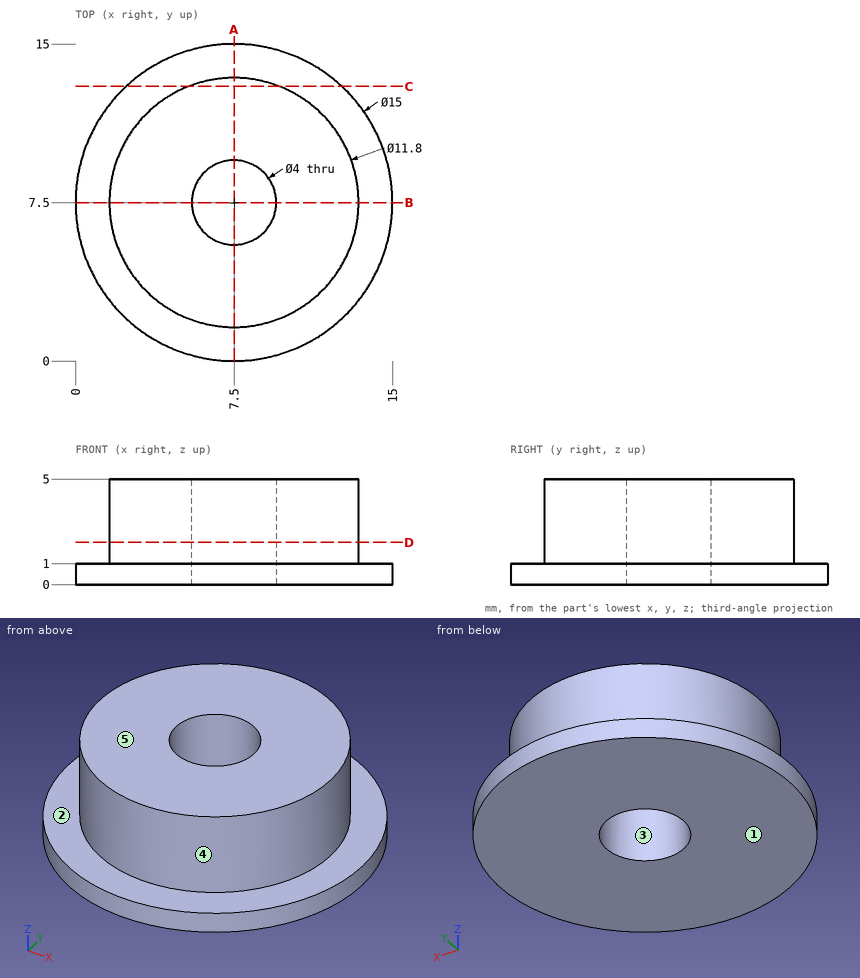
For this review, use the dimensioned drawing (mm, ordinates from the lowest corner) and the shaded views. A direction names the side the tool comes from. Coordinates: 2 decimals unless noted, no trailing zeros. Loops run counter-clockwise (first coordinate to the right, second up) from the corner with the lowest first, then second, coordinate; pieces in that order, holes last. Notation, with made-up numbers: (55.25, 64) -> (112.25, 64) arc R22 ccw to (112.25, 92) -> close; hole circle Ø6 at (79, -24.75). An arc over 180 degrees is marked (long way). Use a Markdown table: item, result. Add a question column.
1. To check wall thickness, follow line 1 (Y direction, x = 7.5, z = 2.75); line 2 (Z direction, x = 11.75, y = 13); line 3 (X direction, y = 5.75, z = 3.1). State the ranges of each line that lie inside material, in increasing order.
2. Draft analysis for pull direction Y (two halves, no side actions). For the marked faces 3, 4 and 5, state which applies: pulls with the +Y half, pulls with the -Y half, needs draft (parallel to the pull), parting line crosses it, or undercut.
3. Add section C-C on y = 13. Write out the cut boundary in (x, z), plus the area to 3 significant figures.
4. Add section A-A on x = 7.5. Write out the cut boundary in (y, z), plus the area to 3 significant figures.
5. Machinability: for the marked faces 1 and 2, which of the approach directions +Z, -Z, +X, -X, +Y, -Y give a long, thin tool a straight path to every point of the face, cutting with its end or side? Answer none if there is none.
6. Add section D-D on z = 2. Write out the cut boundary in (x, y).
7. Clearance check with flat-ended pins moving along their axes: pin 1 Ø1.5 at (y, z) = (6.5, 2.5) entering from -X; pin 2 Ø1.5 at (x, z) = (12, 0.5) entering from +Y; pin 3 Ø3.5 at (x, y) = (7.5, 7.5) entering from -Z. State where each tip first meets the part, or that it passes through.
Returned:
| question | item | result |
|---|---|---|
| 1 | line 1 | y = 1.6 to 5.5, 9.5 to 13.4 |
| 1 | line 2 | z = 0 to 1 |
| 1 | line 3 | x = 1.87 to 6.53, 8.47 to 13.13 |
| 2 | face 3 | undercut |
| 2 | face 4 | parting line crosses it |
| 2 | face 5 | needs draft |
| 3 | outline | (2.4, 0) -> (12.6, 0) -> (12.6, 1) -> (9.64, 1) -> (9.64, 5) -> (5.36, 5) -> (5.36, 1) -> (2.4, 1) -> close |
| 3 | area | 27.3 mm² |
| 4 | outline | (0, 0) -> (5.5, 0) -> (5.5, 5) -> (1.6, 5) -> (1.6, 1) -> (0, 1) -> close; (9.5, 0) -> (15, 0) -> (15, 1) -> (13.4, 1) -> (13.4, 5) -> (9.5, 5) -> close |
| 4 | area | 42.2 mm² |
| 5 | face 1 | -Z, +X, -X, +Y, -Y |
| 5 | face 2 | +Z |
| 6 | outline | circle Ø11.8 at (7.5, 7.5); hole circle Ø4 at (7.5, 7.5) |
| 7 | pin 1 | stops at x = 1.61 |
| 7 | pin 2 | stops at y = 14 |
| 7 | pin 3 | passes through |
